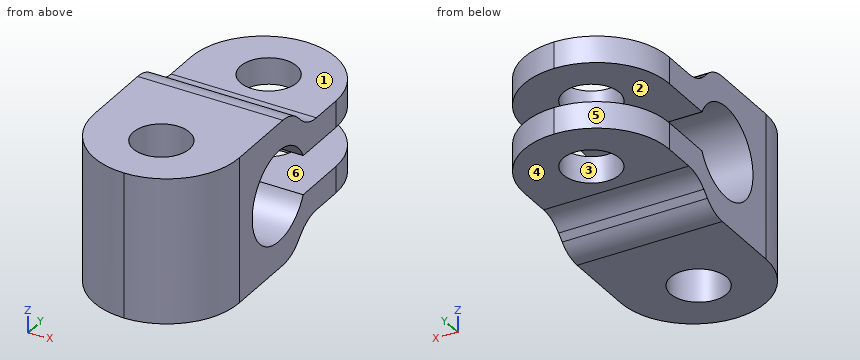
```python
from build123d import *

# Parameters (mm, degrees)
SKETCH_1_W          = 8
SKETCH_1_H          = 17
EXTRUDE_2_DEPTH     = 8
FILLET_2_R          = 4
SKETCH_2_R          = 1.55
CUT_EXTRUDE_1_DEPTH = 8
SKETCH_3_R          = 2.5
CUT_EXTRUDE_2_DEPTH = 8
CUT_EXTRUDE_4_DEPTH = 8
CUT_EXTRUDE_5_DEPTH = 8
FILLET_3_R          = 2


with BuildPart() as part:
    # 草图1 → 凸台-拉伸2 (new body)
    with BuildSketch(Plane.XY):
        with Locations((-4, 8.5)):
            Rectangle(SKETCH_1_W, SKETCH_1_H)
    extrude(amount=EXTRUDE_2_DEPTH)

    # 圆角2
    fillet_2_edges = [part.edges().sort_by_distance(p)[0] for p in [
        (0, 0, 4),
        (-8, 0, 4),
        (0, 17, 4),
        (-8, 17, 4),
    ]]
    fillet(fillet_2_edges, radius=FILLET_2_R - 0.0001)  # a hair under: the kernel refuses the full size

    # 草图2 → 切除-拉伸1 (cut)
    with BuildSketch(Plane.XY.offset(8)):
        with Locations((-4, 13.5)):
            Circle(SKETCH_2_R)
        with Locations((-4, 3.5)):
            Circle(SKETCH_2_R)
    extrude(amount=-CUT_EXTRUDE_1_DEPTH, mode=Mode.SUBTRACT)

    # 草图3 → 切除-拉伸2 (cut)
    with BuildSketch(Plane.ZY.offset(8)):
        with Locations((4, 7.7)):
            Circle(SKETCH_3_R)
    extrude(amount=-CUT_EXTRUDE_2_DEPTH, mode=Mode.SUBTRACT)

    # 草图4 → 切除-拉伸4 (cut)
    with BuildSketch(Plane.ZY.offset(8)):
        with BuildLine():
            Line((2.921520253, 9.955411589), (2.921520253, 17))
            Line((2.921520253, 17), (5.078479747, 17))
            Line((5.078479747, 17), (5.078479747, 9.955411589))
            Line((5.078479747, 9.955411589), (5.078479747, 9.786617836))
            ThreePointArc((5.078479747, 9.786617836), (4, 10.033067636), (2.921520253, 9.786617836))
            Line((2.921520253, 9.786617836), (2.921520253, 9.955411589))
        make_face()
    extrude(amount=-CUT_EXTRUDE_4_DEPTH, mode=Mode.SUBTRACT)

    # 草图5 → 切除-拉伸5 (cut)
    with BuildSketch(Plane.ZY.offset(8)):
        Polygon((0, 8.869306394), (1.460760126, 10.369306394), (1.460760126, 17), (0, 17), align=None)
        Polygon((8, 17), (8, 8.869306394), (6.539239874, 10.369306394), (6.539239874, 17), align=None)
    extrude(amount=-CUT_EXTRUDE_5_DEPTH, mode=Mode.SUBTRACT)

    # 圆角3
    fillet_3_edges = [part.edges().sort_by_distance(p)[0] for p in [
        (-4, 10.369306394, 6.539239874),
        (-4, 8.869306394, 8),
        (-4, 8.869306394, 0),
        (-4, 10.369306394, 1.460760126),
    ]]
    fillet(fillet_3_edges, radius=FILLET_3_R)


solid = part.part
```
Geometry check sheet. Reference: the model listing, model coordinates, mm. Face numbers are marked on the shaded views. A direction names the side the tool comes from. Round coordinates to 2 decimals unless told otherwise and drop trailing zeros. Order: outer loops, then holes, each group sorted by start corner. A loop starts at its lowest first (then second) coordinate and runs counter-clockwise, first axis right, second up. Notation, with made-up numbers: (54, -23) - (80, -23) arc R22 ccw to (80, -7) - close; hole circle Ø6 at (50, -30). An arc over 180 degrees is marked (long way). Use a Markdown table: item, result. Add a question column.
1) Thickness scan on line 1 along Z through (x, y) = (-2.5, 11.75); line 2 along Y through (x, z) = (-3, 5.75); line 3 along Y through (x, z) = (-4, 1.8). Record the ranges inside material, lowest first.
2) Section check C-C (y = 13.5). Record the cut outline in (x, z).
3) Set-up check for the marked faces 1, 2 and 3: record each of +Z, -Z, +X, -X, +Y, -Y from which the full face is reachable in a straight line by a thin tool's end or side.
4) Section check B-B (y = 7.7). Record the cut outline in (x, z).
5) Gauge pin test, flat ends, axial feed: P1, Ø3, axis at y = 15, z = 2, coming from the +X side; P2, Ø3, axis at x = -6, y = 15.5, coming from the +Z side; P3, Ø2.5, axis at x = -4, y = 3.5, coming from the +Z side; P4, Ø3, axis at x = -3, y = 15.5, coming from the -Z side. Record the tip position at first contact, or that the pin passes through.
6) Section check A-A (z = 6). Count the separate pieces of the cut face and the enclosed holes in it, then the cut area to 3 significant figures.
7) Mould release check, pull along Z, two halves, no side actions. Record for the marked faces 4, 5 and 6: released by +Z, released by -Z, zero draft, split by the parting line, or undercut.
Established:
| question | item | result |
|---|---|---|
| 1 | line 1 | 1.46 to 2.92, 5.08 to 6.54 |
| 1 | line 2 | 0.13 to 2.32, 4.68 to 5.91, 9.49 to 12.32, 14.68 to 16.87 |
| 1 | line 3 | 0 to 1.95, 5.05 to 6.51, 8.89 to 11.95, 15.05 to 17 |
| 2 | outline | (-7.97, 1.46) - (-5.55, 1.46) - (-5.55, 2.92) - (-7.97, 2.92) - close; (-7.97, 5.08) - (-5.55, 5.08) - (-5.55, 6.54) - (-7.97, 6.54) - close; (-2.45, 1.46) - (-0.03, 1.46) - (-0.03, 2.92) - (-2.45, 2.92) - close; (-2.45, 5.08) - (-0.03, 5.08) - (-0.03, 6.54) - (-2.45, 6.54) - close |
| 3 | face 1 | +Z, +X, -X, +Y |
| 3 | face 2 | +X, -X, +Y |
| 3 | face 3 | +Z, -Z |
| 4 | outline | (-8, 0) - (0, 0) - (0, 1.5) - (-8, 1.5) - close; (-8, 6.5) - (0, 6.5) - (0, 8) - (-8, 8) - close |
| 5 | P1 | x = -0.03 |
| 5 | P2 | z = 6.54 |
| 5 | P3 | through |
| 5 | P4 | z = 1.46 |
| 6 | separate pieces | 2 |
| 6 | enclosed holes | 2 |
| 6 | area | 83.2 mm2 |
| 7 | face 4 | released by -Z |
| 7 | face 5 | zero draft |
| 7 | face 6 | undercut |
